For this review, take the finished solid that the model builds, in its own axes (mm). Face numbers are marked on the shaded views. Round coordinates to 2 decimals unless told otherwise and drop trailing zeros. Order: outer loops, then holes, each group sorted by start corner. A loop starts at its lowest first (then second) coordinate and runs counter-clockwise, first axis right, second up. Notation, with made-up numbers: (52, 22) - (61, 22) arc R24 cw to (61, 55) - close; hole circle Ø11 at (57, 15.25). An arc over 180 degrees is marked (long way). One line per question, with ' | ' between items.
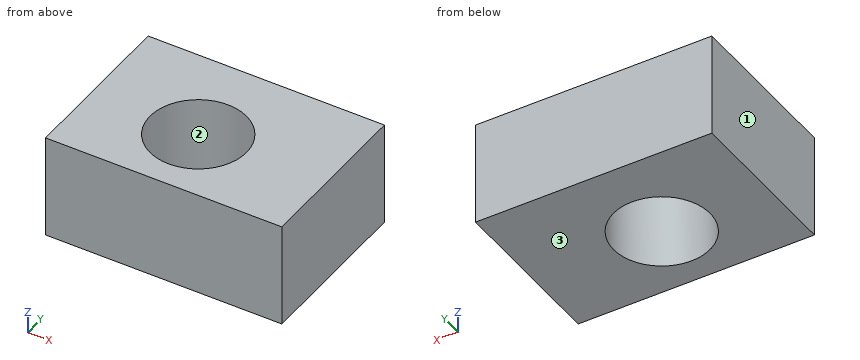
```python
from build123d import *

# Parameters (mm, degrees)
F0_W      = 66.6496
F0_H      = 46.9646
F2_DEPTH  = 29.464
F1_R      = 13.6144
F3_DEPTH  = 48.514
F3_FACE_R = 13.6144
F4_DEPTH  = 84.836


with BuildPart() as f2:
    # F0 (on Top) → F2 (new body)
    with BuildSketch(Plane.XY):
        with Locations((2.836652, 3.065012)):
            Rectangle(F0_W, F0_H)
    extrude(amount=-F2_DEPTH)

    # F1 (on Top) → F3 (join)
    with BuildSketch(Plane.XY):
        Circle(F1_R)
    extrude(amount=-F3_DEPTH)

    # F3_face (on face) → F4 (cut)
    with BuildSketch(Plane(origin=(0, 0, -48.514), x_dir=(1, 0, 0), z_dir=(0, 0, -1))):
        Circle(F3_FACE_R)
    extrude(amount=-F4_DEPTH, mode=Mode.SUBTRACT)


solid = f2.part
```
(1) We need section A-A on x = 0. State the section outline as (y, z) points.
Output values:
outline: (-20.42, -29.46) - (-13.61, -29.46) - (-13.61, 0) - (-20.42, 0) - close; (13.61, -29.46) - (26.55, -29.46) - (26.55, 0) - (13.61, 0) - close
(2) Mouldability with a two-part tool opening along X and no side actions: class the marked faces 1, 2 and 3 as released by +X, released by -X, zero draft, split by the parting line, or undercut.
Output values:
face 1: released by -X | face 2: undercut | face 3: zero draft
(3) We need section C-C on z = -9.75. State the section outline as (x, y) points, plus the area to 3 significant figures.
Output values:
outline: (-30.49, -20.42) - (36.16, -20.42) - (36.16, 26.55) - (-30.49, 26.55) - close; hole circle Ø27.23 at (0, 0) | area: 2,550 mm^2
(4) We need section B-B on y = -9. State the section outline as (x, z) points.
Output values:
outline: (-30.49, -29.46) - (-10.22, -29.46) - (-10.22, 0) - (-30.49, 0) - close; (10.22, -29.46) - (36.16, -29.46) - (36.16, 0) - (10.22, 0) - close
(5) For probe 1 along X at (y, z) = (0, -20.5); probe 2 along Y at (x, z) = (0, -13.5); probe 3 along Y at (x, z) = (8.5, -13.5), list the stretches that pass through material, from the lowest coordinate up. Write a range as [from, to].
Output values:
probe 1: [-30.49, -13.61], [13.61, 36.16] | probe 2: [-20.42, -13.61], [13.61, 26.55] | probe 3: [-20.42, -10.63], [10.63, 26.55]
